Autodesk Inventor part; units mm, degrees
ref_plane "YZ Plane" through (0, 0, 0) normal (1, 0, 0) x (0, 1, 0)
ref_plane "XZ Plane" through (0, 0, 0) normal (0, 1, 0) x (-1, 0, 0)
ref_plane "XY Plane" through (0, 0, 0) normal (0, 0, 1) x (1, 0, 0)
sketch "Эскиз1" plane through (0, 0, 0) normal (0, 0, 1) x (1, 0, 0)
  line L0 (0, 0) -> (29.4445, 0)
  line L1 (0, 47.5) -> (3, 47.5)
  line L2 (0, 47.5) -> (0, 44.5)
  line L3 (0, 44.5) -> (3, 44.5)
  line L4 (3, 47.5) -> (3, 54)
  line L5 (3, 54) -> (9, 54)
  line L6 (9, 54) -> (9, 50)
  line L7 (9, 50) -> (13, 50)
  line L8 (13, 50) -> (13, 37.2933)
  line L9 (13, 37.2933) -> (13, 31)
  line L10 (13, 31) -> (11, 31)
  line L11 (11, 31) -> (11, 40)
  line L12 (11, 40) -> (3, 40)
  line L13 (3, 40) -> (3, 44.5)
  dimension "d2" = 62
  dimension "d3" = 100
  dimension "d5" = 6
  dimension "d6" = 89
  dimension "d7" = 80
  dimension "d8" = 8
  dimension "d9" = 0
  dimension "d10" = 13
  dimension "d15" = 3
  dimension "d16" = 3
  dimension "d17" = 108
revolve "Вращение1" add sketch "Эскиз1" angle 360 about axis through (0, 0, 0) along (1, 0, 0)
chamfer "Фаска1" distance 1 angle 45 1 edges at (13, -50, 0)
properties part number "Крышка правая" material "Сталь, углеродистая"
Read the model definition and answer for the solid it produces. Units are mm, in the model's axes. A direction names the side the tool comes from. Coordinates: 2 decimals unless noted, no trailing zeros. Loops run counter-clockwise (first coordinate to the right, second up) from the corner with the lowest first, then second, coordinate; pieces in that order, holes last.
(1) Flat-ended cylindrical pins translate along their axes: pin 1 Ø6 at (x, y) = (5, -27) entering from +Z; pin 2 Ø10 at (y, z) = (24.5, 27.5) entering from -X; pin 3 Ø6 at (x, y) = (5, -36) entering from +Z. Find the tip coordinate at first contact, or state that the pin passes through.
Solution:
pin 1: stops at z = 48.37
pin 2: stops at x = 3
pin 3: stops at z = 42.74
(2) The mould has two halves that part along Z. Classify faces 1 (the face through (0, -14.3, 42.4)), 2 (the face through (6.94, -8.67, 39.05)), 3 (the face through (10.52, 47.69, 15.02)): released by +Z, released by -Z, zero draft, split by the parting line, or undercut.
Solution:
face 1: zero draft
face 2: undercut
face 3: split by the parting line
(3) The part is cut by section C-C (x = 7). Determine the outline of the cut face in (y, z).
Solution:
outline: circle Ø108 at (0, 0); hole circle Ø80 at (0, 0)
(4) The part is cut by section A-A (z = 0). Determine the outline of the cut face in (x, y).
Solution:
outline: (0, -47.5) - (3, -47.5) - (3, -54) - (9, -54) - (9, -50) - (12, -50) - (13, -49) - (13, -31) - (11, -31) - (11, -40) - (3, -40) - (3, -44.5) - (0, -44.5) - close; (0, 44.5) - (3, 44.5) - (3, 40) - (11, 40) - (11, 31) - (13, 31) - (13, 49) - (12, 50) - (9, 50) - (9, 54) - (3, 54) - (3, 47.5) - (0, 47.5) - close
(5) A tool of negligible diameter and unlimited length cuts with its end or side. For faces 4 (the face through (11, 21, -24)), 5 (the face through (6.042, -11.706, -52.716)), 6 (the face through (9, 48, -16)), from which of +Z, -Z, +X, -X, +Y, -Y can it reach the whole face along a straight path? Write none if from no direction.
Solution:
face 4: -X
face 5: +X, -X
face 6: +X
(6) Consider line 1 along Z through (x, y) = (2.1, 0); line 2 along Z through (x, y) = (11.5, 0); line 3 along X through (y, z) = (-28.5, 45.5). Determine where each line is inside the solid, lowest interval first.
Solution:
line 1: z = -47.5 to -44.5, 44.5 to 47.5
line 2: z = -50 to -31, 31 to 50
line 3: x = 3 to 9
